Read the model definition and answer for the solid it produces. Units are mm, in the model's axes. A direction names the side the tool comes from. Give positions to 0.01 mm unless a question says otherwise; leave off trailing zeros. Order: outer loops, then holes, each group sorted by start corner. A loop starts at its lowest first (then second) coordinate and runs counter-clockwise, first axis right, second up.
Item 1: The mould has two halves that part along Z. Classify faces 4 (the face through (56.1, 4.93, 28.21)), 5 (the face through (65.03, 5, 16)), 6 (the face through (-51, 5, 35.359)): +Z half, -Z half, draft (parallel to the pull), parting line (faces both ways), or undercut.
Item 2: A cutting plane is placed at A-A (y = 6). State how many separate pieces and enclosed holes the cut face has, plus the area to 3 significant figures.
Item 3: Find the intervals of material crossed by line 1 along Z through (x, y) = (35, 1); line 2 along Z through (x, y) = (36, 9); line 3 along Z through (x, y) = (-7, 7.75), in increasing order.
Item 4: Which of the six approach directions +Z, -Z, +X, -X, +Y, -Y give full straight-line access (tool end or side, diameter ignored) to faces 1 (the face through (-26.853, 4.93, 33.567)), 2 (the face through (4, 5, 7.211)), 3 (the face through (43.6, 4.93, 3.21))?
Item 5: A cutting plane is placed at B-B (x = 23). Write down the section's boundary in (y, z), plus the area to 3 significant figures.
Item 6: Given pin 1 Ø5 at (x, y) = (11.5, 5.5) entering from -Z; pin 2 Ø5 at (x, y) = (34.5, 8.5) entering from -Z, each flat-ended and moving along its own axis, determine where each tip first touches the part or whether it passes through.
from build123d import *

# Parameters (mm, degrees)
SKETCH1_R           = 3
BOSS_EXTRUDE1_DEPTH = 10
CHAMFER1_SIZE       = 5


with BuildPart() as part:
    # Sketch1 → Boss-Extrude1 (new body)
    with BuildSketch(Plane(origin=(0, 0, 0), x_dir=(1, 0, 0), z_dir=(0, 1, 0))):
        Polygon((-26.18056889, 2.640536741), (-16.329229088, -7.210803061), (24.381205478, -7.210803061), (34.23254528, 2.640536741), (65.030497816, 2.640536741), (65.030497816, -35.359463259), (34.23254528, -35.359463259), (24.381205478, -25.508123456), (-16.329229088, -25.508123456), (-26.18056889, -35.359463259), (-70.969502184, -35.359463259), (-70.969502184, 2.640536741), align=None)
        with Locations(Location((-65.969502184, -3.859463259, 0), (0, 0, 270))):
            Circle(SKETCH1_R, mode=Mode.SUBTRACT)
        with Locations(Location((-40.969502184, -3.859463259, 0), (0, 0, 270))):
            Circle(SKETCH1_R, mode=Mode.SUBTRACT)
        with Locations(Location((-40.969502184, -28.859463259, 0), (0, 0, 270))):
            Circle(SKETCH1_R, mode=Mode.SUBTRACT)
        with Locations(Location((-65.969502184, -28.859463259, 0), (0, 0, 270))):
            Circle(SKETCH1_R, mode=Mode.SUBTRACT)
        with Locations(Location((-28.469502184, -28.859463259, 0), (0, 0, 270))):
            Circle(SKETCH1_R, mode=Mode.SUBTRACT)
        with Locations(Location((-53.469502184, -3.859463259, 0), (0, 0, 270))):
            Circle(SKETCH1_R, mode=Mode.SUBTRACT)
        with Locations(Location((-53.469502184, -28.859463259, 0), (0, 0, 270))):
            Circle(SKETCH1_R, mode=Mode.SUBTRACT)
        with Locations(Location((-28.469502184, -3.859463259, 0), (0, 0, 270))):
            Circle(SKETCH1_R, mode=Mode.SUBTRACT)
        with Locations(Location((34.030497816, -3.859463259, 0), (0, 0, 270))):
            Circle(SKETCH1_R, mode=Mode.SUBTRACT)
        with Locations(Location((59.030497816, -28.859463259, 0), (0, 0, 270))):
            Circle(SKETCH1_R, mode=Mode.SUBTRACT)
        with Locations(Location((59.030497816, -3.859463259, 0), (0, 0, 270))):
            Circle(SKETCH1_R, mode=Mode.SUBTRACT)
        with Locations(Location((34.030497816, -28.859463259, 0), (0, 0, 270))):
            Circle(SKETCH1_R, mode=Mode.SUBTRACT)
        with Locations(Location((46.530497816, -28.859463259, 0), (0, 0, 270))):
            Circle(SKETCH1_R, mode=Mode.SUBTRACT)
        with Locations(Location((46.530497816, -3.859463259, 0), (0, 0, 270))):
            Circle(SKETCH1_R, mode=Mode.SUBTRACT)
    extrude(amount=BOSS_EXTRUDE1_DEPTH)

    # Chamfer1
    chamfer1_edges = [part.edges().sort_by_distance(p)[0] for p in [
        (-26.18056889, 5, -2.640536741),
        (34.23254528, 5, -2.640536741),
        (34.23254528, 5, 35.359463259),
        (-26.18056889, 5, 35.359463259),
    ]]
    chamfer(chamfer1_edges, length=CHAMFER1_SIZE)


solid = part.part
Response values:
1. face 4: undercut
1. face 5: draft
1. face 6: +Z half
2. separate pieces: 1
2. enclosed holes: 14
2. area: 3,740 mm2
3. line 1: z = -0.89 to 1.02, 6.7 to 26.02, 31.7 to 33.61
3. line 2: z = -1.3 to 1.6, 6.12 to 26.6, 31.12 to 34.02
3. line 3: z = 7.21 to 25.51
4. face 1: +Z, +Y, -Y
4. face 2: -Z, +Y, -Y
4. face 3: +Y, -Y
5. outline: (0, 7.21) - (10, 7.21) - (10, 25.51) - (0, 25.51) - close
5. area: 183 mm2
6. pin 1: stops at z = 7.21
6. pin 2: stops at z = -1.72
